Work out the finished part from the listing and answer in its coordinate system (mm). Face numbers are marked on the shaded views. A direction names the side the tool comes from. Give positions to 0.01 mm unless a question says otherwise; leave off trailing zeros. Write each loop counter-clockwise with the first axis right and the second up, starting at its lowest first coordinate (ties: lowest second). Pieces come first, ordered by that corner, then holes. Notation, with made-up numbers: (61.25, -19.5) - (87.25, -19.5) arc R15 cw to (87.25, -3.5) - close; hole circle Ø4 at (-4.5, 45). An arc over 180 degrees is marked (long way). Write item = value, one per line.
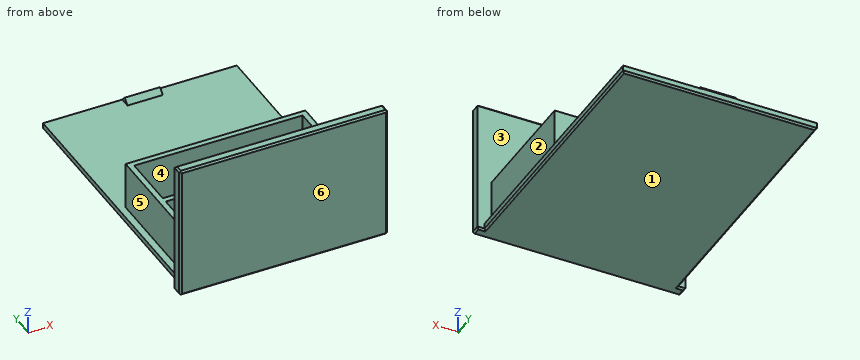
Autodesk Inventor part; units mm, degrees
ref_plane "YZ Plane" through (0, 0, 0) normal (1, 0, 0) x (0, 1, 0)
ref_plane "XZ Plane" through (0, 0, 0) normal (0, 1, 0) x (-1, 0, 0)
ref_plane "XY Plane" through (0, 0, 0) normal (0, 0, 1) x (1, 0, 0)
sketch "Sketch1" plane through (0, 0, 0) normal (0, 0, 1) x (1, 0, 0)
  line L0 (0, 0) -> (55, 0)
  line L1 (55, 0) -> (55, 80)
  line L2 (55, 80) -> (0, 80)
  line L3 (0, 80) -> (0, 0)
  dimension "d0" = 55
  dimension "d1" = 80
extrude "Base" add sketch "Sketch1" along normal blind 2
sketch "Sketch2" plane through (0, 0, 2) normal (0, 0, 1) x (1, 0, 0)
  line L0 (55, 0) -> (55, 80)
  line L1 (0, 80) -> (0, 0)
  line L2 (-2, 0) -> (57, 0)
  line L3 (57, 0) -> (57, 3)
  line L4 (57, 3) -> (-2, 3)
  line L5 (-2, 3) -> (-2, 0)
  dimension "d4" = 3
  dimension "d5" = 2
  dimension "d6" = 2
extrude "Back" add sketch "Sketch2" along normal blind 36.5 and the other way blind 2
sketch "Sketch6" plane through (0, 0, 2) normal (0, 0, 1) x (1, 0, 0)
  line L0 (0, 80) -> (0, 3)
  line L1 (0, 3) -> (55, 3)
  line L2 (55, 3) -> (55, 80)
  line L3 (2, 3) -> (53, 3)
  line L4 (53, 3) -> (53, 38)
  line L5 (53, 38) -> (2, 38)
  line L6 (2, 38) -> (2, 3)
  point P0 (0, 0)
  dimension "d29" = 35
  dimension "d30" = 2
  dimension "d31" = 2
extrude "Box" add sketch "Sketch6" along normal blind 13.5
chamfer "Chamfer3" distance 0.5 angle 45 8 edges at (0, 41.5, 0) (27.5, 80, 0) (55, 41.5, 0) (-1, 3, 0) (-2, 1.5, 0) (27.5, 0, 0) (57, 1.5, 0) (56, 3, 0)
chamfer "Chamfer4" distance 0.5 angle 45 3 edges at (-2, 0, 19.5) (27.5, 0, 38.5) (57, 0, 19.5)
chamfer "Chamfer5" distance 0.5 angle 45 3 edges at (-2, 1.75, 38.5) (27.5, 3, 38.5) (57, 1.75, 38.5)
sketch "Sketch7" plane through (0, 0, 15.5) normal (0, 0, 1) x (1, 0, 0)
  line L0 (53, 3) -> (2, 3)
  line L1 (53, 3) -> (53, 38)
  line L2 (53, 38) -> (2, 38)
  line L3 (2, 38) -> (2, 3)
  line L4 (3.6, 3) -> (51.4, 3)
  line L5 (51.4, 3) -> (51.4, 18.9)
  line L6 (51.4, 18.9) -> (3.6, 18.9)
  line L7 (3.6, 18.9) -> (3.6, 3)
  line L8 (51.4, 36.4) -> (3.6, 36.4)
  line L9 (3.6, 36.4) -> (3.6, 20.5)
  line L10 (3.6, 20.5) -> (51.4, 20.5)
  line L11 (51.4, 20.5) -> (51.4, 36.4)
  point P0 (0, 0)
  dimension "d44" = 1.6
  dimension "d45" = 1.6
  dimension "d46" = 1.6
  dimension "d47" = 1.6
  dimension "d48" = 1.6
  dimension "d49" = 1.6
  dimension "d50" = 15.9
  dimension "d51" = 15.9
extrude "Box inside" cut sketch "Sketch7" against normal blind 13.5 contours L0 L7 L6 L5 | L11 L10 L9 L8
sketch "Sketch8" plane through (0, 0, 2) normal (0, 0, 1) x (1, 0, 0)
  line L0 (55, 3) -> (55, 80)
  line L1 (55, 80) -> (0, 80)
  line L2 (0, 80) -> (0, 3)
  line L3 (22.5, 80) -> (32.5, 80)
  line L4 (32.5, 80) -> (32.5, 77.1)
  line L5 (32.5, 77.1) -> (22.5, 77.1)
  line L6 (22.5, 77.1) -> (22.5, 80)
  point P0 (0, 0)
  dimension "d63" = 22.5
  dimension "d64" = 22.5
  dimension "d65" = 10
  dimension "d66" = 2.9
extrude "Extrusion8" add sketch "Sketch8" along normal blind 1.5
chamfer "Chamfer9" distance 1.5 angle 45 1 edges at (27.5, 77.1, 3.5)
chamfer "Chamfer10" distance 1.4 angle 45 1 edges at (27.5, 80, 3.5)
equation "\"d31\" = d30"
equation "\"d45\" = d44"
equation "\"d46\" = d45"
equation "\"d47\" = d46"
equation "\"d48\" = d44"
equation "\"d49\" = d44"
equation "\"d64\" = d63"
properties part number "BOTTOM"
1. A tool of negligible diameter and unlimited length cuts with its end or side. For the marked faces 1 and 2, from which of +Z, -Z, +X, -X, +Y, -Y can it reach the whole face along a straight path? Write none if from no direction.
Solution:
face_1 = -Z, +X, -X, +Y, -Y
face_2 = +Z, +X, +Y
2. Given pin 1 (7 mm diameter, centred on y = 11, z = 7, fed in from +X); pin 2 (1.5 mm diameter, centred on x = 4.5, y = 39.5, fed in from +Z); pin 3 (1 mm diameter, centred on x = 29, z = 25, fed in from +Y), each flat-ended and moving along its own axis, determine where each tip first touches the part or whether it passes through.
Solution:
pin_1 = 53
pin_2 = 2
pin_3 = 3
3. Find section D-D, the plane z = 28.5. Give the vertices of the cut face in (x, y).
Solution:
outline = (-2, 0.5) - (-1.5, 0) - (56.5, 0) - (57, 0.5) - (57, 3) - (-2, 3) - close
4. Straight lines are drawn through the part: line 1 (Y direction, x = 42.5, z = 4); line 2 (X direction, y = 22.5, z = 6); line 3 (Y direction, x = 41.5, z = 20.5). For each, find the intervals that lie inside material, in ascending order.
Solution:
line_1 = 0 to 3, 18.9 to 20.5, 36.4 to 38
line_2 = 2 to 3.6, 51.4 to 53
line_3 = 0 to 3
5. Find section C-C, the plane y = 10. Give the vertices of the cut face in (x, z), then the cut area to 3 significant figures.
Solution:
outline = (0, 0.5) - (0.5, 0) - (54.5, 0) - (55, 0.5) - (55, 2) - (53, 2) - (53, 15.5) - (51.4, 15.5) - (51.4, 2) - (3.6, 2) - (3.6, 15.5) - (2, 15.5) - (2, 2) - (0, 2) - close
area = 153 mm^2
6. For a pull along Y with two mould halves and no side action, classify the marked faces 3, 4, 5 and 6 as pulls with the +Y half, pulls with the -Y half, needs draft (parallel to the pull), parting line crosses it, or undercut.
Solution:
face_3 = undercut
face_4 = undercut
face_5 = needs draft
face_6 = pulls with the -Y half
7. Find section A-A, the plane z = 14. Give the vertices of the cut face in (x, y).
Solution:
outline = (-2, 0.5) - (-1.5, 0) - (56.5, 0) - (57, 0.5) - (57, 3) - (53, 3) - (53, 38) - (2, 38) - (2, 3) - (-2, 3) - close; hole (3.6, 3) - (51.4, 3) - (51.4, 18.9) - (3.6, 18.9) - close; hole (3.6, 20.5) - (51.4, 20.5) - (51.4, 36.4) - (3.6, 36.4) - close
